```python
from build123d import *

# Parameters (mm, degrees)
SKETCH1_R           = 22
BOSS_EXTRUDE1_DEPTH = 9
SHELL2_T            = -1
CUT_EXTRUDE1_DEPTH  = 5
CUT_EXTRUDE2_DEPTH  = 5
SKETCH24_W          = 2.319445398
SKETCH24_H          = 3.83352781
CUT_EXTRUDE3_DEPTH  = 5
SKETCH25_W          = 10.887577437
SKETCH25_H          = 4.540244535
BOSS_EXTRUDE2_DEPTH = 4
SKETCH26_R          = 1.75
CUT_EXTRUDE4_DEPTH  = 5
SKETCH27_W          = 9.75823175
SKETCH27_H          = 4.730401218
BOSS_EXTRUDE3_DEPTH = 4
SKETCH28_R          = 1.75
CUT_EXTRUDE5_DEPTH  = 6


with BuildPart() as part:
    # Sketch1 → Boss-Extrude1 (new body)
    with BuildSketch(Plane.XY):
        Circle(SKETCH1_R)
    extrude(amount=BOSS_EXTRUDE1_DEPTH)

    # Shell2
    shell2_openings = [part.faces().sort_by_distance(p)[0] for p in [
        (0, 0, 0),
    ]]
    offset(amount=SHELL2_T, openings=shell2_openings, kind=Kind.INTERSECTION)

    # Sketch23 → Cut-Extrude1 (cut)
    with BuildSketch(Plane(origin=(0, 0, 8), x_dir=(-1, 0, 0), z_dir=(0, 0, -1))):
        with BuildLine():
            Line((-3.104308234, -18.303704212), (-3.104308234, 18.303704212))
            ThreePointArc((-3.104308234, 18.303704212), (-2.460017846, 18.9479946), (-1.815727458, 18.303704212))
            Line((-1.815727458, 18.303704212), (-1.815727458, -18.303704212))
            ThreePointArc((-1.815727458, -18.303704212), (-2.460017846, -18.9479946), (-3.104308234, -18.303704212))
        make_face()
        with BuildLine():
            Line((-6.032900908, -17.307982703), (-6.032900908, 17.307982703))
            ThreePointArc((-6.032900908, 17.307982703), (-5.271466813, 18.069416798), (-4.510032718, 17.307982703))
            Line((-4.510032718, 17.307982703), (-4.510032718, -17.307982703))
            ThreePointArc((-4.510032718, -17.307982703), (-5.271466813, -18.069416798), (-6.032900908, -17.307982703))
        make_face()
        with BuildLine():
            Line((-8.610062461, -16.546548608), (-8.610062461, 16.546548608))
            ThreePointArc((-8.610062461, 16.546548608), (-7.965772073, 17.190838996), (-7.321481685, 16.546548608))
            Line((-7.321481685, 16.546548608), (-7.321481685, -16.546548608))
            ThreePointArc((-7.321481685, -16.546548608), (-7.965772073, -17.190838996), (-8.610062461, -16.546548608))
        make_face()
        with BuildLine():
            Line((-10.894364747, -15.667970806), (-10.894364747, 15.667970806))
            ThreePointArc((-10.894364747, 15.667970806), (-10.367218066, 16.195117487), (-9.840071384, 15.667970806))
            Line((-9.840071384, 15.667970806), (-9.840071384, -15.667970806))
            ThreePointArc((-9.840071384, -15.667970806), (-10.367218066, -16.195117487), (-10.894364747, -15.667970806))
        make_face()
        with BuildLine():
            Line((-13.4715263, -13.617955934), (-13.4715263, 13.617955934))
            ThreePointArc((-13.4715263, 13.617955934), (-12.827235912, 14.262246322), (-12.182945524, 13.617955934))
            Line((-12.182945524, 13.617955934), (-12.182945524, -13.617955934))
            ThreePointArc((-12.182945524, -13.617955934), (-12.827235912, -14.262246322), (-13.4715263, -13.617955934))
        make_face()
        with BuildLine():
            Line((-16.16583156, -11.040794381), (-16.16583156, 11.040794381))
            ThreePointArc((-16.16583156, 11.040794381), (-15.462969318, 11.743656623), (-14.760107077, 11.040794381))
            Line((-14.760107077, 11.040794381), (-14.760107077, -11.040794381))
            ThreePointArc((-14.760107077, -11.040794381), (-15.462969318, -11.743656623), (-16.16583156, -11.040794381))
        make_face()
        with BuildLine():
            Line((-18.567277553, -5.945043128), (-18.567277553, 5.945043128))
            ThreePointArc((-18.567277553, 5.945043128), (-18.040130871, 6.472189809), (-17.51298419, 5.945043128))
            Line((-17.51298419, 5.945043128), (-17.51298419, -5.945043128))
            ThreePointArc((-17.51298419, -5.945043128), (-18.040130871, -6.472189809), (-18.567277553, -5.945043128))
        make_face()
    extrude(amount=-CUT_EXTRUDE1_DEPTH, mode=Mode.SUBTRACT)

    # Sketch22 → Cut-Extrude2 (cut)
    with BuildSketch(Plane(origin=(0, 0, 8), x_dir=(-1, 0, 0), z_dir=(0, 0, -1))):
        with BuildLine():
            Line((-0.527146681, -18.59656348), (-0.527146681, 18.59656348))
            ThreePointArc((-0.527146681, 18.59656348), (0, 19.123710161), (0.527146681, 18.59656348))
            Line((0.527146681, 18.59656348), (0.527146681, -18.59656348))
            ThreePointArc((0.527146681, -18.59656348), (0, -19.123710161), (-0.527146681, -18.59656348))
        make_face()
        with BuildLine():
            Line((1.581440044, -18.127988652), (1.581440044, 18.127988652))
            ThreePointArc((1.581440044, 18.127988652), (2.284302286, 18.830850893), (2.987164527, 18.127988652))
            Line((2.987164527, 18.127988652), (2.987164527, -18.127988652))
            ThreePointArc((2.987164527, -18.127988652), (2.284302286, -18.830850893), (1.581440044, -18.127988652))
        make_face()
        with BuildLine():
            Line((4.275745304, -17.42512641), (4.275745304, 17.42512641))
            ThreePointArc((4.275745304, 17.42512641), (4.978607546, 18.127988652), (5.681469787, 17.42512641))
            Line((5.681469787, 17.42512641), (5.681469787, -17.42512641))
            ThreePointArc((5.681469787, -17.42512641), (4.978607546, -18.127988652), (4.275745304, -17.42512641))
        make_face()
        with BuildLine():
            Line((7.321481685, -16.780836022), (7.321481685, 16.780836022))
            ThreePointArc((7.321481685, 16.780836022), (7.965772073, 17.42512641), (8.610062461, 16.780836022))
            Line((8.610062461, 16.780836022), (8.610062461, -16.780836022))
            ThreePointArc((8.610062461, -16.780836022), (7.965772073, -17.42512641), (7.321481685, -16.780836022))
        make_face()
        with BuildLine():
            Line((10.074358798, -15.023680417), (10.074358798, 15.023680417))
            ThreePointArc((10.074358798, 15.023680417), (10.718649187, 15.667970806), (11.362939575, 15.023680417))
            Line((11.362939575, 15.023680417), (11.362939575, -15.023680417))
            ThreePointArc((11.362939575, -15.023680417), (10.718649187, -15.667970806), (10.074358798, -15.023680417))
        make_face()
        with BuildLine():
            Line((12.710092205, -13.266524813), (12.710092205, 13.266524813))
            ThreePointArc((12.710092205, 13.266524813), (13.237238886, 13.793671494), (13.764385568, 13.266524813))
            Line((13.764385568, 13.266524813), (13.764385568, -13.266524813))
            ThreePointArc((13.764385568, -13.266524813), (13.237238886, -13.793671494), (12.710092205, -13.266524813))
        make_face()
        with BuildLine():
            Line((14.701535223, -10.455075846), (14.701535223, 10.455075846))
            ThreePointArc((14.701535223, 10.455075846), (15.228681905, 10.982222527), (15.755828586, 10.455075846))
            Line((15.755828586, 10.455075846), (15.755828586, -10.455075846))
            ThreePointArc((15.755828586, -10.455075846), (15.228681905, -10.982222527), (14.701535223, -10.455075846))
        make_face()
        with BuildLine():
            Line((16.810121948, -6.999336491), (16.810121948, 6.999336491))
            ThreePointArc((16.810121948, 6.999336491), (17.278696776, 7.467911319), (17.747271604, 6.999336491))
            Line((17.747271604, 6.999336491), (17.747271604, -6.999336491))
            ThreePointArc((17.747271604, -6.999336491), (17.278696776, -7.467911319), (16.810121948, -6.999336491))
        make_face()
    extrude(amount=-CUT_EXTRUDE2_DEPTH, mode=Mode.SUBTRACT)

    # Sketch24 → Cut-Extrude3 (cut)
    with BuildSketch(Plane(origin=(22, 0, 0), x_dir=(0, 0, -1), z_dir=(1, 0, 0))):
        with Locations((-4.159722699, 1.916763905)):
            Rectangle(SKETCH24_W, SKETCH24_H)
    extrude(amount=-CUT_EXTRUDE3_DEPTH, mode=Mode.SUBTRACT)

    # Sketch25 → Boss-Extrude2 (add)
    with BuildSketch(Plane(origin=(0, 0, 0), x_dir=(-1, 0, 0), z_dir=(0, 0, -1))):
        with Locations((-0.56321323, 23.434146639)):
            Rectangle(SKETCH25_W, SKETCH25_H)
    extrude(amount=-BOSS_EXTRUDE2_DEPTH)

    # Sketch26 → Cut-Extrude4 (cut)
    with BuildSketch(Plane(origin=(0, 0, 0), x_dir=(-1, 0, 0), z_dir=(0, 0, -1))):
        with Locations((-2.366226378, 23.54446207)):
            Circle(SKETCH26_R)
    extrude(amount=-CUT_EXTRUDE4_DEPTH, mode=Mode.SUBTRACT)

    # Sketch27 → Boss-Extrude3 (add)
    with BuildSketch(Plane(origin=(0, 0, 0), x_dir=(-1, 0, 0), z_dir=(0, 0, -1))):
        with Locations((-0.307450986, -23.745086582)):
            Rectangle(SKETCH27_W, SKETCH27_H)
    extrude(amount=-BOSS_EXTRUDE3_DEPTH)

    # Sketch28 → Cut-Extrude5 (cut)
    with BuildSketch(Plane(origin=(0, 0, 0), x_dir=(-1, 0, 0), z_dir=(0, 0, -1))):
        with Locations((0, -23.598199513)):
            Circle(SKETCH28_R)
    extrude(amount=-CUT_EXTRUDE5_DEPTH, mode=Mode.SUBTRACT)


solid = part.part
```
Design review of the part built by this model. Coordinates are the model's own, in mm. A direction names the side the tool comes from. Coordinates: 2 decimals unless noted, no trailing zeros. Write each loop counter-clockwise with the first axis right and the second up, starting at its lowest first coordinate (ties: lowest second). Pieces come first, ordered by that corner, then holes.
1) Add section A-A (z = 1.75). Write out the cut boundary in (x, y), plus the area to 3 significant figures.
2) To check wall thickness, follow L1, parallel to Y at x = 0, z = 3; L2, parallel to Z at x = -11, y = 16; L3, parallel to Y at x = -12, z = 7.75. State the ranges of each line that lie inside material, in increasing order.
3) Insertion check: pin 1 (0.8 mm diameter, centred on y = -1.5, z = 8.5, fed in from +X); pin 2 (3 mm diameter, centred on x = -7, z = 6.5, fed in from +Y); pin 3 (3 mm diameter, centred on y = 10, z = 3.5, fed in from +X); pin 4 (2 mm diameter, centred on x = 2.37, y = 23.54, fed in from +Z) (1 decimal). Each pin has a flat end and moves straight along its axis. Give the tip position at first contact, or say it passes through.
4) Add section B-B (y = -2). State how many separate pieces and enclosed holes the cut face has, plus the area to 3 significant figures.
5) Machinability: for faces 4 (the cylindrical face through (20.03, 6.31, 3.94)), 5 (the flat face through (6.007, 23, 2)), 6 (the flat face through (5.187, -24, 2)), which of the approach directions +Z, -Z, +X, -X, +Y, -Y give a long, thin tool a straight path to every point of the face, cutting with its end or side? Answer none if there is none.
6) Mouldability with a two-part tool opening along Y and no side actions: class faces 1 (the flat face through (1, 25.704, 2)), 2 (the cylindrical face through (0.228, -21.863, 2.291)), 3 (the flat face through (0.6, 24.5, 4)) as +Y half, -Y half, draft (parallel to the pull), parting line (faces both ways), or undercut.
Check result:
1. outline: (-4.88, 21.45) arc R22 ccw to (-4.57, -21.52) - (-4.57, -26.11) - (5.19, -26.11) - (5.19, -21.38) arc R22 ccw to (6.01, 21.16) - (6.01, 25.7) - (-4.88, 25.7) - close; hole circle Ø42 at (0, 0); hole circle Ø3.5 at (0, -23.6); hole circle Ø3.5 at (2.37, 23.54)
1. area: 201 mm2
2. L1: y = -26.11 to -25.35, -21.85 to -21, 21 to 25.7
2. L2: z = 8 to 9
2. L3: y = -18.44 to -17.23, 17.23 to 18.44
3. pin 1: stops at x = 21.97
3. pin 2: stops at y = 21.3
3. pin 3: stops at x = 20.29
3. pin 4: passes through
4. separate pieces: 16
4. enclosed holes: 0
4. area: 41.5 mm2
5. face 4: -Z
5. face 5: +Z, -Z, +X, +Y
5. face 6: +Z, -Z, +X, -Y
6. face 1: +Y half
6. face 2: undercut
6. face 3: draft
